Design review of the part built by this model. Coordinates are the model's own, in mm. Face numbers are marked on the shaded views. A direction names the side the tool comes from. Give positions to 0.01 mm unless a question says otherwise; leave off trailing zeros. Order: outer loops, then holes, each group sorted by start corner. A loop starts at its lowest first (then second) coordinate and runs counter-clockwise, first axis right, second up. Notation, with made-up numbers: (-23.5, 31) -> (-18.5, 31) arc R20 cw to (-18.5, 56) -> close; hole circle Ø1 at (79.5, -10). An arc over 180 degrees is marked (long way). Return JSON: item names as keys, results as strings.
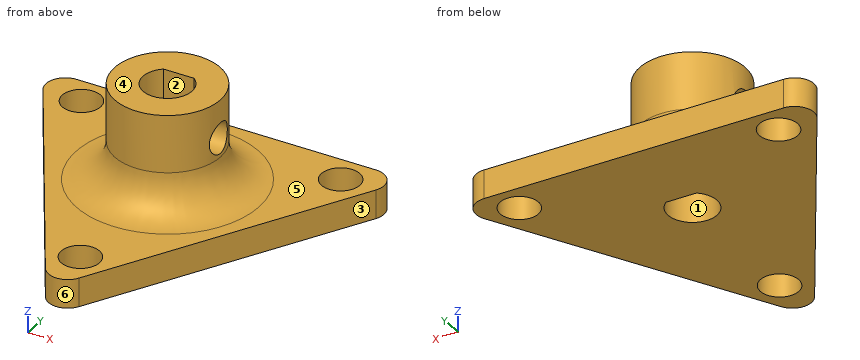
```python
from build123d import *

# Parameters (mm, degrees)
SKETCH1_R               = 2.000000038
SKETCH1_R_2             = 1.999999864
SKETCH1_R_3             = 1.999999855
BOSS_EXTRUDE1_DEPTH     = 3
SKETCH2_R               = 5.5
BOSS_EXTRUDE2_DEPTH     = 10
CUT_EXTRUDE1_DEPTH      = 30.235355095
CUT_EXTRUDE1_DEPTH_BACK = 30.235355095
FILLET1_R               = 2
FILLET2_R               = 4
CUT_EXTRUDE2_DEPTH      = 28.078088376
CUT_EXTRUDE2_DEPTH_BACK = 28.078088376
SKETCH4_R               = 1.6


with BuildPart() as part:
    # Sketch1 → Boss-Extrude1 (new body)
    with BuildSketch(Plane.XY):
        Polygon((-19.186339187, 14.630551858), (18.813660813, 14.630551858), (1.3e-07, -17.821065516), align=None)
        with Locations((-13.429805086, 11.630551858)):
            Circle(SKETCH1_R, mode=Mode.SUBTRACT)
        with Locations((13.429804917, 11.630551858)):
            Circle(SKETCH1_R_2, mode=Mode.SUBTRACT)
        with Locations((8.5e-08, -11.630551858)):
            Circle(SKETCH1_R_3, mode=Mode.SUBTRACT)
    extrude(amount=BOSS_EXTRUDE1_DEPTH)

    # Sketch2 → Boss-Extrude2 (add)
    with BuildSketch(Plane.XY.offset(3)):
        with Locations((0, 3.880551858)):
            Circle(SKETCH2_R)
    extrude(amount=BOSS_EXTRUDE2_DEPTH)

    # Sketch3 → Cut-Extrude1 (cut, two sides: drawn at the far end of the back side and taken through both)
    with BuildSketch(Plane.XY.offset(13).offset(-CUT_EXTRUDE1_DEPTH_BACK)):
        with BuildLine():
            Line((-1.581929202, 5.880551858), (1.581929202, 5.880551858))
            ThreePointArc((1.581929202, 5.880551858), (0, 1.330551858), (-1.581929202, 5.880551858))
        make_face()
    extrude(amount=CUT_EXTRUDE1_DEPTH + CUT_EXTRUDE1_DEPTH_BACK, mode=Mode.SUBTRACT)

    # Fillet1
    fillet1_edges = [part.edges().sort_by_distance(p)[0] for p in [
        (-19.186339187, 14.630551858, 1.5),
        (18.813660813, 14.630551858, 1.5),
        (1.3e-07, -17.821065516, 1.5),
    ]]
    fillet(fillet1_edges, radius=FILLET1_R)

    # Fillet2
    fillet2_edges = [part.edges().sort_by_distance(p)[0] for p in [
        (-5.5, 3.880551858, 3),
    ]]
    fillet(fillet2_edges, radius=FILLET2_R)

    # Sketch4 → Cut-Extrude2 (cut, two sides: drawn at the far end of the back side and taken through both)
    with BuildSketch(Plane(origin=(0, 0, 0), x_dir=(0, 0, -1), z_dir=(1, 0, 0)).offset(-CUT_EXTRUDE2_DEPTH_BACK)):
        with Locations((-9, 3.880551858)):
            Circle(SKETCH4_R)
    extrude(amount=CUT_EXTRUDE2_DEPTH + CUT_EXTRUDE2_DEPTH_BACK, mode=Mode.SUBTRACT)


solid = part.part
```
Item 1: Add section C-C (x = -15). Give the boundary of the cut face in (y, z), plus the area to 3 significant figures.
Result set:
{"outline": "(7.55, 0) -> (10.39, 0) -> (10.39, 3) -> (7.55, 3) -> close; (12.87, 0) -> (14.63, 0) -> (14.63, 3) -> (12.87, 3) -> close", "area": "13.8 mm^2"}
Item 2: Wall thickness on L1, parallel to Y at x = 0, z = 1; L2, parallel to Z at x = -5.5, y = -5; L3, parallel to Y at x = 2, z = 8.25: over which ranges is each line inside the solid? List them lowest first. Write a range as [from, to].
Result set:
{"L1": "y = [-15.86, -13.63], [-9.63, 1.33], [5.88, 14.63]", "L2": "z = [0, 3]", "L3": "y = [-1.24, 2.3], [5.46, 9]"}
Item 3: Add section B-B (x = 0). Give the boundary of the cut face in (y, z).
Result set:
{"outline": "(-15.86, 0) -> (-13.63, 0) -> (-13.63, 3) -> (-15.86, 3) -> close; (-9.63, 0) -> (1.33, 0) -> (1.33, 13) -> (-1.62, 13) -> (-1.62, 7) arc R4 cw to (-5.62, 3) -> (-9.63, 3) -> close; (5.88, 0) -> (14.63, 0) -> (14.63, 3) -> (13.38, 3) arc R4 cw to (9.38, 7) -> (9.38, 13) -> (5.88, 13) -> close"}
Item 4: Add section D-D (y = 12.5). Give the number of separate pieces and of enclosed holes in the cut face, plus the area to 3 significant figures.
Result set:
{"separate pieces": "3", "enclosed holes": "0", "area": "83.8 mm^2"}
Item 5: For pin 1 (3 mm diameter, centred on x = 0, y = -11.63, fed in from +Z); pin 2 (1 mm diameter, centred on x = -8.5, y = 5.5, fed in from -Z); pin 3 (4 mm diameter, centred on y = 7.5, z = 6.5, fed in from +X); pin 4 (2 mm diameter, centred on y = 3, z = 5, fed in from +X), all flat-tipped, find the tip position at first contact; note any pin that passes through.
Result set:
{"pin 1": "passes through", "pin 2": "stops at z = 0", "pin 3": "stops at x = 5.6", "pin 4": "stops at x = 6.8"}
Item 6: Machinability: for the marked faces 5 and 6, which of the approach directions +Z, -Z, +X, -X, +Y, -Y give a long, thin tool a straight path to every point of the face, cutting with its end or side? Answer none if there is none.
Result set:
{"face 5": "+Z", "face 6": "+Z, -Z, -Y"}
Item 7: Add section A-A (z = 8). Give the boundary of the cut face in (x, y), plus the area to 3 significant figures.
Result set:
{"outline": "(-5.36, 2.63) arc R5.5 ccw to (5.36, 2.63) -> (2.22, 2.63) arc R2.55 cw to (-2.22, 2.63) -> close; (-5.36, 5.13) -> (-2.22, 5.13) arc R2.55 cw to (-1.58, 5.88) -> (1.58, 5.88) arc R2.55 cw to (2.22, 5.13) -> (5.36, 5.13) arc R5.5 ccw to start", "area": "60.8 mm^2"}
Item 8: Mouldability with a two-part tool opening along Y and no side actions: class the marked faces 1, 2, 3 and 4 as released by +Y, released by -Y, zero draft, split by the parting line, or undercut.
Result set:
{"face 1": "undercut", "face 2": "undercut", "face 3": "released by -Y", "face 4": "zero draft"}
